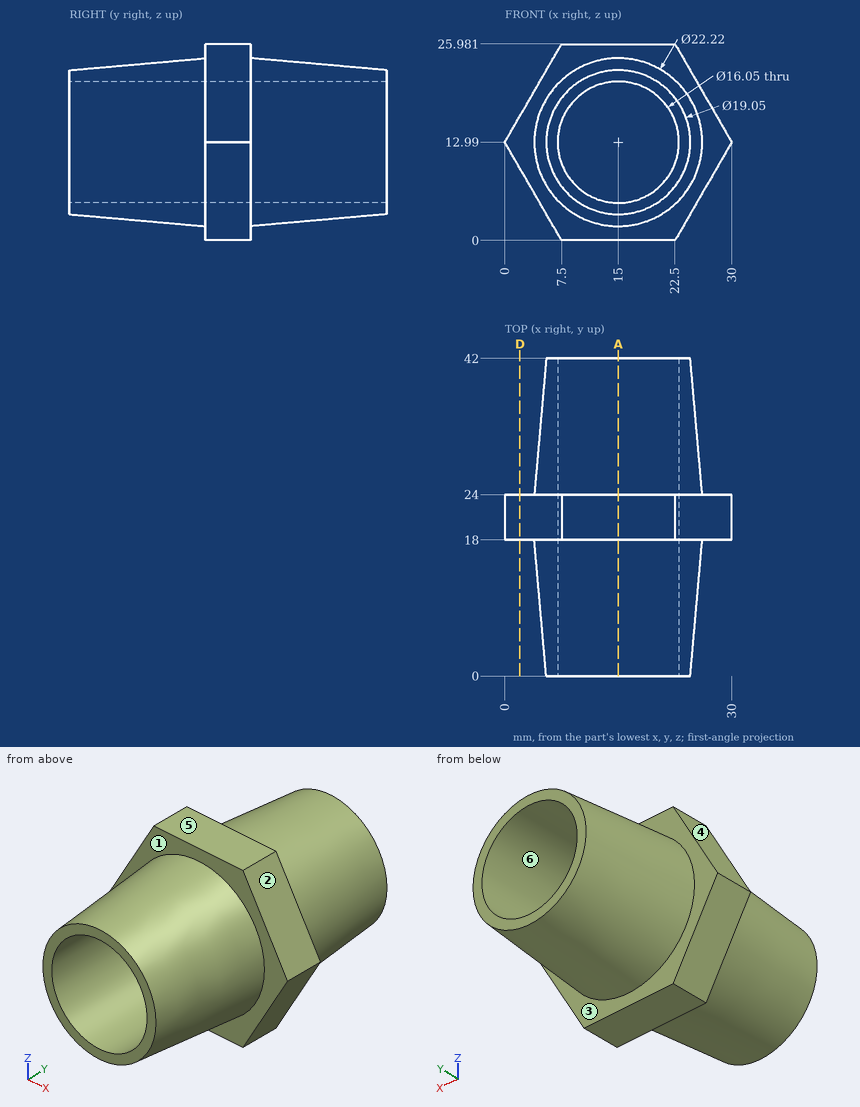
Input: dimensioned drawing with shaded views. Units: mm. Origin: part minimum x, y, z. A direction names the side the tool comes from. Give positions to 0.01 mm unless a question says otherwise; leave off trailing zeros. Order: outer loops, then holes, each group sorted by start corner. A loop starts at its lowest first (then second) coordinate and runs counter-clockwise, first axis right, second up. Notation, with made-up numbers: (68.5, 35) -> (93.5, 35) arc R19 ccw to (93.5, 55) -> close; hole circle Ø7 at (24, 48.25). An arc over 180 degrees is marked (long way). Write item = value, one per line.
Item 1: Contact query for flat-ended pins moving along their axis: pin 1 (12 mm diameter, centred on x = 13.5, y = 5.5, fed in from -Z); pin 2 (8 mm diameter, centred on x = 23, z = 22, fed in from -Y); pin 3 (4 mm diameter, centred on x = 22, y = 35.5, fed in from -Z); pin 4 (2 mm diameter, centred on x = 3.5, z = 19, fed in from -Y). Output: stop coordinate, or through.
Check result:
pin_1 = 2.47
pin_2 = 0
pin_3 = 4.2
pin_4 = 18
Item 2: Mould query, pull axis X, two halves, no side actions, for the marked faces 4, 5 and 6. Classes: +X half, -X half, draft (parallel to the pull), parting line (faces both ways), or undercut.
Check result:
face_4 = -X half
face_5 = draft
face_6 = undercut
Item 3: Ray query, probe 1 along Z at (x, y) = (15, 20.5) (1 decimal); probe 2 along X at (y, z) = (23.5, 18); probe 3 along X at (y, z) = (26, 20.25) (1 decimal). Return the intervals inside material, ascending.
Check result:
probe_1 = 0 to 5, 21 to 26
probe_2 = 2.89 to 8.73, 21.27 to 27.11
probe_3 = 6.8 to 11.6, 18.4 to 23.2
Item 4: Section query D-D (x = 2). Output: boundary loops of the cut face in (y, z) (1 decimal).
Check result:
outline = (18, 9.5) -> (24, 9.5) -> (24, 16.5) -> (18, 16.5) -> close
Item 5: Set-up query: the marked faces 1, 2 and 3. Return all of +Z, -Z, +X, -X, +Y, -Y with unobstructed straight access to the full face (end or side cutting, diameter ignored); none if empty.
Check result:
face_1 = -Y
face_2 = +Z, +X, +Y, -Y
face_3 = +Y
Item 6: Section query A-A (x = 15). Output: boundary loops of the cut face in (y, z) (1 decimal).
Check result:
outline = (0, 3.5) -> (18, 1.9) -> (18, 0) -> (24, 0) -> (24, 1.9) -> (42, 3.5) -> (42, 5) -> (0, 5) -> close; (0, 21) -> (42, 21) -> (42, 22.5) -> (24, 24.1) -> (24, 26) -> (18, 26) -> (18, 24.1) -> (0, 22.5) -> close
